```python
from build123d import *

# Parameters (mm, degrees)
EXTRUDE_1_DEPTH          = 1.85
SKETCH_2_W               = 0.7
SKETCH_2_H               = 1.6
SKETCH_2_W_2             = 1.02
SKETCH_2_H_2             = 1
EXTRUDE_2_DEPTH          = 0.1
SKETCH_3_R               = 0.4
EXTRUDE_3_DEPTH          = 0.6
CUT_EXTRUDE_1_DEPTH      = 12.62835328
CUT_EXTRUDE_1_DEPTH_BACK = 7
SKETCH_4_W               = 11.1
SKETCH_4_H               = 0.95
FILLET_1_R               = 0.1
FILLET_2_R               = 0.1


with BuildPart() as part:
    # 스케치1 → 보스-돌출1 (new body)
    with BuildSketch(Plane(origin=(0, 0, 0), x_dir=(1, 0, 0), z_dir=(0, 1, 0))):
        Polygon((2.66, -6.15), (5.16, -6.85), (7.86, -6.85), (7.86, 6.15), (6.84, 6.15), (6.84, 7.65), (-6.84, 7.65), (-6.84, -6.15), align=None)
    extrude(amount=EXTRUDE_1_DEPTH)

    # 스케치2 → 보스-돌출2 (add)
    with BuildSketch(Plane(origin=(0, 0, 0), x_dir=(1, 0, 0), z_dir=(0, 1, 0))):
        with Locations((8.21, -2.45)):
            Rectangle(SKETCH_2_W, SKETCH_2_H)
        with Locations((7.35, 7.15)):
            Rectangle(SKETCH_2_W_2, SKETCH_2_H_2)
        with Locations((-7.19, 7.15)):
            Rectangle(SKETCH_2_W, SKETCH_2_H_2)
        with Locations((-7.19, -2.45)):
            Rectangle(SKETCH_2_W, SKETCH_2_H)
    extrude(amount=EXTRUDE_2_DEPTH)

    # 스케치3 → 보스-돌출3 (add)
    with BuildSketch(Plane.XZ):
        with Locations(Location((-4.95, 2.85, 0), (0, 0, 90))):
            Circle(SKETCH_3_R)
        with Locations(Location((3.05, 2.85, 0), (0, 0, 90))):
            Circle(SKETCH_3_R)
    extrude(amount=EXTRUDE_3_DEPTH)

    # 스케치4 → 컷-돌출1 (cut, two sides: drawn at the far end of the back side and taken through both)
    with BuildSketch(Plane.XY.offset(-CUT_EXTRUDE_1_DEPTH_BACK)):
        with Locations((-0.49, 1.275)):
            Rectangle(SKETCH_4_W, SKETCH_4_H)
    extrude(amount=CUT_EXTRUDE_1_DEPTH + CUT_EXTRUDE_1_DEPTH_BACK, mode=Mode.SUBTRACT)

    # 필렛1
    fillet_1_edges = [part.edges().sort_by_distance(p)[0] for p in [
        (-4.95, -0.6, 2.45),
        (3.05, -0.6, 2.45),
    ]]
    fillet(fillet_1_edges, radius=FILLET_1_R)

    # 필렛2
    fillet_2_edges = [part.edges().sort_by_distance(p)[0] for p in [
        (6.84, 0.1, -7.15),
        (7.86, 0.1, 2.45),
        (-6.84, 0.1, -7.15),
        (-6.84, 0.1, 2.45),
    ]]
    fillet(fillet_2_edges, radius=FILLET_2_R)


solid = part.part
```
Geometry: final body of the model. Coordinates: model frame, mm. A direction names the side the tool comes from. Give positions to 0.01 mm unless a question says otherwise; leave off trailing zeros. Write each loop counter-clockwise with the first axis right and the second up, starting at its lowest first coordinate (ties: lowest second). Pieces come first, ordered by that corner, then holes.
1. Section query B-B, the plane y = 1.15. Return loops of the section in (x, z).
2. Section query C-C, the plane x = -4.95. Return loops of the section in (y, z), then the cut area to 3 significant figures.
3. Reachability of faces 1 (the flat face through (0, 1, -7.65)), 2 (the flat face through (-6.04, 1, -1)), 3 (the flat face through (-2.2, 0.5, 6.15)) from +Z, -Z, +X, -X, +Y, -Y: full face, straight path, thin tool, end or side. Return the list, or none.
4. Line query: probe 1 along X at (y, z) = (1.3, -2.5); probe 2 along Z at (x, y) = (4.75, 1.35); probe 3 along Y at (x, z) = (7.25, 0.75). Output: solid intervals per line, ascending.
5. Pin query (flat end, axial travel): P1, Ø8, axis at x = -4, z = -2, coming from the -Y side; P2, Ø0.5, axis at y = 1.5, z = 1, coming from the +X side. Return the tip coordinate at first contact, or that it passes through.
6. Section query D-D, the plane z = -0.5. Return loops of the section in (x, y), then the cut area to 4 significant figures.
7. Draft query along Y for faces 4 (the flat face through (-6.84, 1, -1)), 5 (the flat face through (0, 0, -1)), 6 (the flat face through (5.06, 1, 0)). Return one class per face: released by +Y, released by -Y, zero draft, split by the parting line, or undercut.
8. Section query A-A, the plane z = 2.85. Return loops of the section in (x, y), then the cut area to 3 significant figures.
Computed:
1. outline: (-6.84, -7.65) - (6.84, -7.65) - (6.84, -6.15) - (7.86, -6.15) - (7.86, 6.85) - (5.16, 6.85) - (5.06, 6.82) - (5.06, -7) - (-6.04, -7) - (-6.04, 6.15) - (-6.84, 6.15) - close
2. outline: (-0.6, 2.55) arc R0.1 ccw to (-0.5, 2.45) - (0, 2.45) - (0, -7.65) - (1.85, -7.65) - (1.85, 6.15) - (1.75, 6.15) - (1.75, -7) - (0.8, -7) - (0.8, 6.15) - (0, 6.15) - (0, 3.25) - (-0.5, 3.25) arc R0.1 ccw to (-0.6, 3.15) - close
2. area: 13.5 mm2
3. face 1: -Z, +X, -X, +Y, -Y
3. face 2: +Z
3. face 3: +Z, -X, +Y, -Y
4. probe 1: x = -6.84 to -6.04, 5.06 to 7.86
4. probe 2: z = -7.65 to -7
4. probe 3: y = 0 to 1.85
5. P1: stops at y = 0
5. P2: stops at x = 7.86
6. outline: (-6.84, 0) - (7.86, 0) - (7.86, 1.85) - (-6.84, 1.85) - close; hole (-6.04, 0.8) - (5.06, 0.8) - (5.06, 1.75) - (-6.04, 1.75) - close
6. area: 16.65 mm2
7. face 4: zero draft
7. face 5: released by -Y
7. face 6: undercut
8. outline: (-7.54, 0) - (-5.35, 0) - (-5.35, -0.5) arc R0.1 ccw to (-5.25, -0.6) - (-4.65, -0.6) arc R0.1 ccw to (-4.55, -0.5) - (-4.55, 0) - (2.65, 0) - (2.65, -0.5) arc R0.1 ccw to (2.75, -0.6) - (3.35, -0.6) arc R0.1 ccw to (3.45, -0.5) - (3.45, 0) - (8.56, 0) - (8.56, 0.1) - (7.96, 0.1) arc R0.1 cw to (7.86, 0.2) - (7.86, 1.85) - (-6.84, 1.85) - (-6.84, 0.2) arc R0.1 cw to (-6.94, 0.1) - (-7.54, 0.1) - close; hole (-6.04, 0.8) - (5.06, 0.8) - (5.06, 1.75) - (-6.04, 1.75) - close
8. area: 17.7 mm2
